Can you work these out from the drawing? Everything is in mm from the part's minimum corner. A direction names the side the tool comes from. Coordinates: 2 decimals unless noted, no trailing zeros. Write each loop counter-clockwise with the first axis right and the second up, starting at its lowest first coordinate (ties: lowest second). Pieces come first, ordered by that corner, then holes. Notation, with made-up numbers: (79, -16) -> (123, -16) arc R19 ccw to (123, 0) -> close; hole circle Ø1 at (-38.5, 80). An arc over 180 degrees is marked (long way). Use CSV: the item, a comma, the result in double quotes. Start each with the question number.
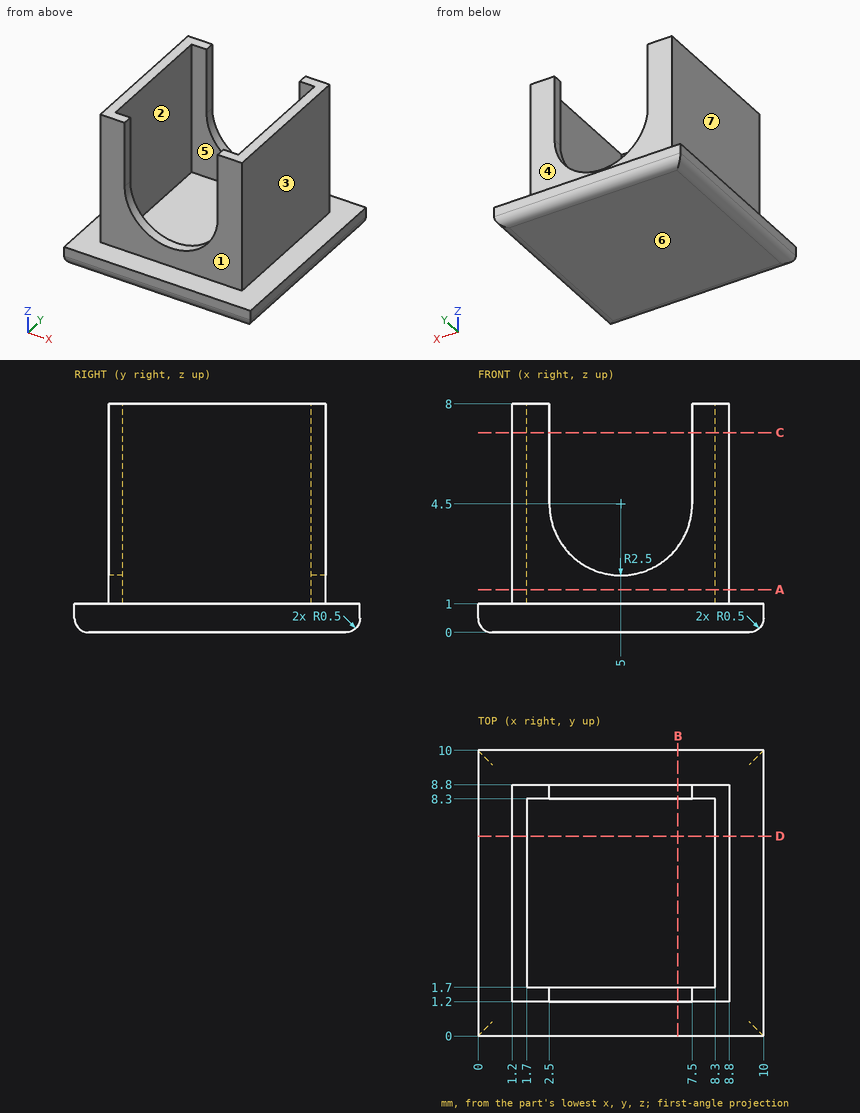
Item 1: I'm going to push flat-ended pins straight in: pin 1 (4 mm diameter, centred on y = 5, z = 2, fed in from +X); pin 2 (0.6 mm diameter, centred on y = 1.5, z = 7, fed in from -X); pin 3 (2 mm diameter, centred on x = 9, z = 2.5, fed in from -Y); pin 4 (0.6 mm diameter, centred on y = 8.5, z = 5.5, fed in from +X). Where does each tip first touch, or does it pass through?
Item 2: I want a section at A-A on z = 1.5. Please give me the cut outline in (x, y), then the cut area to 3 significant figures.
Item 3: I want a section at C-C on z = 7. Please give me the cut outline in (x, y), then the cut area to 3 significant figures.
Item 4: I want a section at D-D on y = 7. Please give me the cut outline in (x, z), then the cut area to 3 significant figures.
Item 5: Which directions (+Z, -Z, +X, -X, +Y, -Y) give clear straight access to the entire face, cutting with the end or side of a thin tool? Please do the marked faces 5, 6 and 7.
Item 6: I want a section at B-B on x = 7. Please give me the cut outline in (y, z).
Item 7: If I drill on line 1 along X through (y, z) = (5.5, 2.25); line 2 along X through (y, z) = (1.5, 6.75), over which ranges is the centre line in solid material (lowest first)?
Item 8: Thinking about a two-plate mould opening in Y: for the marked faces 1, 2, 3 and 4, which applies, +Y half, -Y half, draft (parallel to the pull), parting line (faces both ways), or undercut?
Geometry says:
1,pin 1,"x = 10"
1,pin 2,"x = 1.2"
1,pin 3,"y = 1.2"
1,pin 4,"x = 8.8"
2,outline,"(1.2, 1.2) -> (8.8, 1.2) -> (8.8, 8.8) -> (1.2, 8.8) -> close; hole (1.7, 1.7) -> (8.3, 1.7) -> (8.3, 8.3) -> (1.7, 8.3) -> close"
2,area,"14.2 mm2"
3,outline,"(1.2, 1.2) -> (2.5, 1.2) -> (2.5, 1.7) -> (1.7, 1.7) -> (1.7, 8.3) -> (2.5, 8.3) -> (2.5, 8.8) -> (1.2, 8.8) -> close; (7.5, 1.2) -> (8.8, 1.2) -> (8.8, 8.8) -> (7.5, 8.8) -> (7.5, 8.3) -> (8.3, 8.3) -> (8.3, 1.7) -> (7.5, 1.7) -> close"
3,area,"9.20 mm2"
4,outline,"(0, 0.5) arc R0.5 ccw to (0.5, 0) -> (9.5, 0) arc R0.5 ccw to (10, 0.5) -> (10, 1) -> (8.8, 1) -> (8.8, 8) -> (8.3, 8) -> (8.3, 1) -> (1.7, 1) -> (1.7, 8) -> (1.2, 8) -> (1.2, 1) -> (0, 1) -> close"
4,area,"16.9 mm2"
5,face 5,"+Z"
5,face 6,"-Z, +X, -X, +Y, -Y"
5,face 7,"+Z, -X, +Y, -Y"
6,outline,"(0, 0.5) arc R0.5 ccw to (0.5, 0) -> (9.5, 0) arc R0.5 ccw to (10, 0.5) -> (10, 1) -> (8.8, 1) -> (8.8, 3) -> (8.3, 3) -> (8.3, 1) -> (1.7, 1) -> (1.7, 3) -> (1.2, 3) -> (1.2, 1) -> (0, 1) -> close"
7,line 1,"1.2 to 1.7, 8.3 to 8.8"
7,line 2,"1.2 to 2.5, 7.5 to 8.8"
8,face 1,"-Y half"
8,face 2,"undercut"
8,face 3,"draft"
8,face 4,"+Y half"
